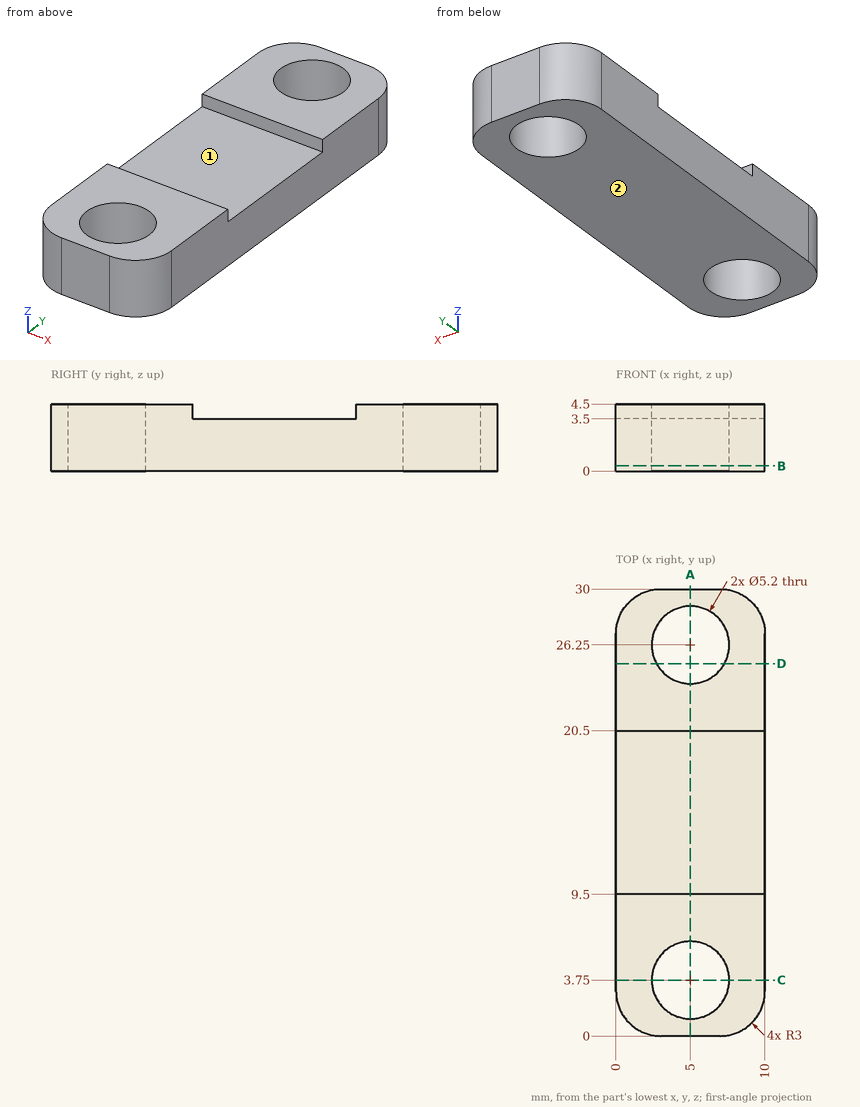
Input: dimensioned drawing with shaded views. Units: mm. Origin: part minimum x, y, z. A direction names the side the tool comes from. Round coordinates to 2 decimals unless told otherwise and drop trailing zeros. Loops run counter-clockwise (first coordinate to the right, second up) from the corner with the lowest first, then second, coordinate; pieces in that order, holes last. Notation, with made-up numbers: (6, -17.5) -> (23, -17.5) arc R19 cw to (23, 11.5) -> close; hole circle Ø3 at (-23, 31). An arc over 180 degrees is marked (long way). Answer as a JSON object with one key per item and string values. Group by question number.
1) Section query D-D on y = 25. Output: boundary loops of the cut face in (x, z), plus the area to 3 significant figures.
2) Section query A-A on x = 5. Output: boundary loops of the cut face in (y, z), plus the area to 3 significant figures.
3) Section query B-B on z = 0.35. Output: boundary loops of the cut face in (x, y).
4) Pin query (flat end, axial travel): pin 1 (0.8 mm diameter, centred on x = 3.5, z = 4, fed in from -Y); pin 2 (4.5 mm diameter, centred on x = 5, y = 26.25, fed in from +Z). Return the tip coordinate at first contact, or that it passes through.
5) Section query C-C on y = 3.75. Output: boundary loops of the cut face in (x, z).
6) Reachability of the marked faces 1 and 2 from +Z, -Z, +X, -X, +Y, -Y: full face, straight path, thin tool, end or side. Return the list, or none.
7) Ray query, L1, parallel to Y at x = 5, z = 2.25; L2, parallel to Y at x = 5, z = 3.6; L3, parallel to X at y = 26.25, z = 1.65. Return the intervals inside material, ascending.
Reply:
{
 "1": {"outline": "(0, 0) -> (2.72, 0) -> (2.72, 4.5) -> (0, 4.5) -> close; (7.28, 0) -> (10, 0) -> (10, 4.5) -> (7.28, 4.5) -> close", "area": "24.5 mm2"},
 "2": {"outline": "(0, 0) -> (1.15, 0) -> (1.15, 4.5) -> (0, 4.5) -> close; (6.35, 0) -> (23.65, 0) -> (23.65, 4.5) -> (20.5, 4.5) -> (20.5, 3.5) -> (9.5, 3.5) -> (9.5, 4.5) -> (6.35, 4.5) -> close; (28.85, 0) -> (30, 0) -> (30, 4.5) -> (28.85, 4.5) -> close", "area": "77.2 mm2"},
 "3": {"outline": "(0, 3) arc R3 ccw to (3, 0) -> (7, 0) arc R3 ccw to (10, 3) -> (10, 27) arc R3 ccw to (7, 30) -> (3, 30) arc R3 ccw to (0, 27) -> close; hole circle Ø5.2 at (5, 3.75); hole circle Ø5.2 at (5, 26.25)"},
 "4": {"pin 1": "stops at y = 0", "pin 2": "passes through"},
 "5": {"outline": "(0, 0) -> (2.4, 0) -> (2.4, 4.5) -> (0, 4.5) -> close; (7.6, 0) -> (10, 0) -> (10, 4.5) -> (7.6, 4.5) -> close"},
 "6": {"face 1": "+Z, +X, -X", "face 2": "-Z, +X, -X, +Y, -Y"},
 "7": {"L1": "y = 0 to 1.15, 6.35 to 23.65, 28.85 to 30", "L2": "y = 0 to 1.15, 6.35 to 9.5, 20.5 to 23.65, 28.85 to 30", "L3": "x = 0 to 2.4, 7.6 to 10"}
}
